Could you check a few things on this drawing? It's one solid part, dimensions in mm from its lowest x, y, z. A direction names the side the tool comes from. Coordinates: 2 decimals unless noted, no trailing zeros. Write each loop counter-clockwise with the first axis right and the second up, starting at its lowest first coordinate (ties: lowest second). Pieces come first, ordered by that corner, then holes.
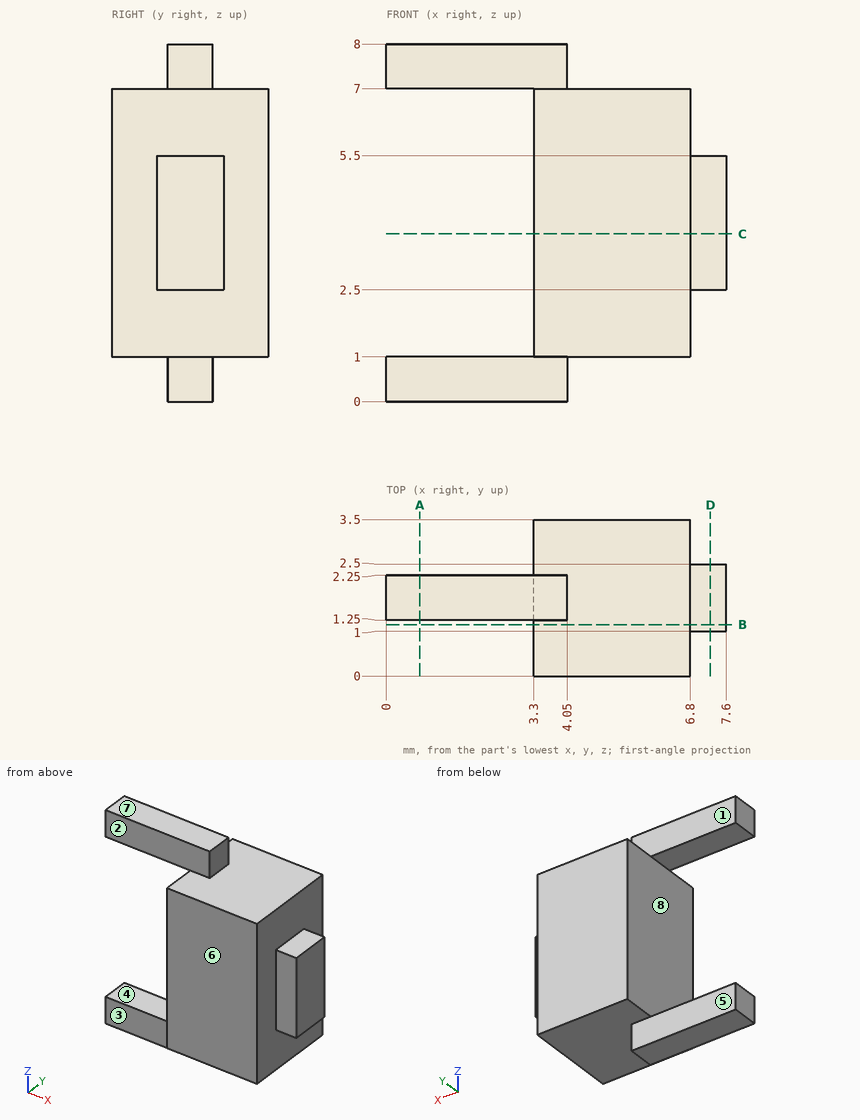
1) Imagine slicing it at B-B on y = 1.15. Please give me the cut outline in (x, z), then the cut area to 3 significant figures.
Values follow:
outline: (3.3, 1) - (6.8, 1) - (6.8, 2.5) - (7.6, 2.5) - (7.6, 5.5) - (6.8, 5.5) - (6.8, 7) - (3.3, 7) - close
area: 23.4 mm2
2) I need wall thicknesses on probe 1 along X at (y, z) = (1.55, 2.75); probe 2 along Z at (x, y) = (6.5, 0.35); probe 3 along X at (y, z) = (1.6, 1.5). Which ranges of each line are inside material? Lowest first, please.
Values follow:
probe 1: x = 3.3 to 7.6
probe 2: z = 1 to 7
probe 3: x = 3.3 to 6.8
3) Will these pins go through, and if not, where does the flat tip stop? pin 1 (1 mm diameter, centred on y = 2.5, z = 7, fed in from +X); pin 2 (0.6 mm diameter, centred on x = 7, y = 1.5, fed in from +Z); pin 3 (0.5 mm diameter, centred on x = 1.5, z = 7.5, fed in from -Y).
Values follow:
pin 1: stops at x = 6.8
pin 2: stops at z = 7
pin 3: stops at y = 1.25
4) Imagine slicing it at C-C on z = 3.75. Please give me the cut outline in (x, y), then the cut area to 4 significant figures.
Values follow:
outline: (3.3, 0) - (6.8, 0) - (6.8, 1) - (7.6, 1) - (7.6, 2.5) - (6.8, 2.5) - (6.8, 3.5) - (3.3, 3.5) - close
area: 13.45 mm2
5) Imagine slicing it at D-D on x = 7.25. Please give me the cut outline in (y, z).
Values follow:
outline: (1, 2.5) - (2.5, 2.5) - (2.5, 5.5) - (1, 5.5) - close
6) On a 3-axis mill with a long thin cutter (end or side, diameter ignored), from which of +Z, -Z, +X, -X, +Y, -Y can I reach the whole of each face in a straight line? I mean the marked faces 1, 2, 3, 4 and 5. Say none if no direction works.
Values follow:
face 1: +Z, +X, -X, +Y
face 2: +Z, +X, -X, -Y
face 3: -Z, +X, -X, -Y
face 4: -X, +Y, -Y
face 5: -Z, +X, -X, +Y
7) Imagine slicing it at A-A on x = 0.75. Please give me the cut outline in (y, z).
Values follow:
outline: (1.25, 0) - (2.25, 0) - (2.25, 1) - (1.25, 1) - close; (1.25, 7) - (2.25, 7) - (2.25, 8) - (1.25, 8) - close
8) We'd pull the mould along Z, two halves only. Please class the marked faces 6, 7 and 8: pulls with the +Z half, pulls with the -Z half, needs draft (parallel to the pull), parting line crosses it, or undercut.
Values follow:
face 6: needs draft
face 7: pulls with the +Z half
face 8: undercut
